from build123d import *

# Parameters (mm, degrees)
ESQUISSE1_W             = 94
ESQUISSE1_H             = 93.807810261
ESQUISSE1_R             = 7
BOSS_EXTRU_1_DEPTH      = 5
ESQUISSE2_R             = 1.5
ENL_V_MAT_EXTRU_1_DEPTH = 67.655832453
ESQUISSE3_R             = 1.5
ENL_V_MAT_EXTRU_2_DEPTH = 10


with BuildPart() as part:
    # Esquisse1 → Boss.-Extru.1 (new body)
    with BuildSketch(Plane.XY):
        with Locations((0, 0.096094869)):
            Rectangle(ESQUISSE1_W, ESQUISSE1_H)
        Circle(ESQUISSE1_R, mode=Mode.SUBTRACT)
    extrude(amount=BOSS_EXTRU_1_DEPTH)

    # Esquisse2 → Enlèv. mat.-Extru.1 (cut, through all)
    with BuildSketch(Plane.XY.offset(5)):
        with Locations((9.5, 0)):
            Circle(ESQUISSE2_R)
        with BuildLine():
            Line((25, 47), (25, 0))
            ThreePointArc((25, 0), (0, -25), (-25, 0))
            Line((-25, 0), (-25, 47))
            Line((-25, 47), (-47, 47))
            Line((-47, 47), (-47, -46.807810261))
            Line((-47, -46.807810261), (47, -46.807810261))
            Line((47, -46.807810261), (47, 47))
            Line((47, 47), (25, 47))
        make_face()
        with Locations((-9.5, 0)):
            Circle(ESQUISSE2_R)
        with Locations((0, 9.5)):
            Circle(ESQUISSE2_R)
        with Locations((0, -9.5)):
            Circle(ESQUISSE2_R)
    extrude(amount=-ENL_V_MAT_EXTRU_1_DEPTH, mode=Mode.SUBTRACT)

    # Esquisse3 → Enlèv. mat.-Extru.2 (cut)
    with BuildSketch(Plane(origin=(0, 47, 0), x_dir=(1, 0, 0), z_dir=(0, 1, 0))):
        with Locations(Location((0, -2.5, 0), (0, 0, 270))):
            Circle(ESQUISSE3_R)
        with Locations(Location((-19, -2.5, 0), (0, 0, 270))):
            Circle(ESQUISSE3_R)
        with Locations(Location((19, -2.5, 0), (0, 0, 270))):
            Circle(ESQUISSE3_R)
    extrude(amount=-ENL_V_MAT_EXTRU_2_DEPTH, mode=Mode.SUBTRACT)


solid = part.part
Here's how the part is built. I have some questions about the finished solid (model axes, mm). A direction names the side the tool comes from. Coordinates: 2 decimals unless noted, no trailing zeros. Order: outer loops, then holes, each group sorted by start corner. A loop starts at its lowest first (then second) coordinate and runs counter-clockwise, first axis right, second up. Notation, with made-up numbers: M -25.5,-0.75 L -5.5,-0.75 A26 cw -5.5,29.25 Z; hole C 89,-26.5 d2. An arc over 180 degrees is marked long. Answer as CSV lines item,"result".
Item 1: If I drill on line 1 (Y direction, x = 0, z = 1.6); line 2 (X direction, y = 45, z = 2.5); line 3 (Y direction, x = -9.5, z = 3.1), over which ranges is the centre line in solid material (lowest first)?
Results found:
line 1,"-25 to -11, -8 to -7, 7 to 8, 11 to 37"
line 2,"-25 to -20.5, -17.5 to -1.5, 1.5 to 17.5, 20.5 to 25"
line 3,"-23.12 to -1.5, 1.5 to 47"
Item 2: For pin 1 (4 mm diameter, centred on x = 0, y = -9.5, fed in from +Z); pin 2 (2.5 mm diameter, centred on x = 19, z = 2.5, fed in from +Y), each with a flat end and sliding along its axis, tell me the tip position at first contact or that it passes through.
Results found:
pin 1,"z = 5"
pin 2,"y = 37"
Item 3: We'd pull the mould along Z, two halves only. Please class faces 3 (the face through (6.466, -2.681, 2.465)), 4 (the face through (19, 37, 2)), 5 (the face through (0, 12, 0)), 6 (the face through (0, 12, 5)): +Z half, -Z half, draft (parallel to the pull), parting line (faces both ways), or undercut.
Results found:
face 3,"draft"
face 4,"undercut"
face 5,"-Z half"
face 6,"+Z half"
Item 4: Imagine slicing it at C-C on z = 1.75. Write out the boundary of the cut face in (x, y).
Results found:
outline,"M -25,0 A25 ccw 25,0 L 25,47 L 20.3,47 L 20.3,37 L 17.7,37 L 17.7,47 L 1.3,47 L 1.3,37 L -1.3,37 L -1.3,47 L -17.7,47 L -17.7,37 L -20.3,37 L -20.3,47 L -25,47 Z; hole C -9.5,0 d3; hole C 0,0 d14; hole C 0,-9.5 d3; hole C 0,9.5 d3; hole C 9.5,0 d3"
Item 5: Imagine slicing it at D-D on x = -9.5. Write out the boundary of the cut face in (y, z), plus the area to 3 significant figures.
Results found:
outline,"M -23.12,0 L -1.5,0 L -1.5,5 L -23.12,5 Z; M 1.5,0 L 47,0 L 47,5 L 1.5,5 Z"
area,"336 mm2"
Item 6: Imagine slicing it at A-A on x = 0. Write out the boundary of the cut face in (y, z), plus the area to 3 significant figures.
Results found:
outline,"M -25,0 L -11,0 L -11,5 L -25,5 Z; M -8,0 L -7,0 L -7,5 L -8,5 Z; M 7,0 L 8,0 L 8,5 L 7,5 Z; M 11,0 L 47,0 L 47,1 L 37,1 L 37,4 L 47,4 L 47,5 L 11,5 Z"
area,"230 mm2"
Item 7: Imagine slicing it at B-B on y = -3. Write out the boundary of the cut face in (x, z).
Results found:
outline,"M -24.82,0 L -6.32,0 L -6.32,5 L -24.82,5 Z; M 6.32,0 L 24.82,0 L 24.82,5 L 6.32,5 Z"
Item 8: On a 3-axis mill with a long thin cutter (end or side, diameter ignored), from which of +Z, -Z, +X, -X, +Y, -Y can I reach the whole of each face in a straight line? I mean faces 1 (the face through (-17.513, 42.07, 2.305)), 2 (the face through (0, 8, 3)). Say none if no direction works.
Results found:
face 1,"+Y"
face 2,"+Z, -Z"
